Model file for the job. Use its own axes, mm. Face numbers are marked on the shaded views. A direction names the side the tool comes from. Round coordinates to 2 decimals unless told otherwise and drop trailing zeros. Order: outer loops, then holes, each group sorted by start corner. A loop starts at its lowest first (then second) coordinate and runs counter-clockwise, first axis right, second up. Notation, with made-up numbers: M 70,0.5 L 91,0.5 A16 ccw 91,30.5 Z; hole C 25.5,14.5 d1. An arc over 180 degrees is marked long. Return JSON: item names as keys, results as strings. Group by question number.
Item 1: Slice it at D-D on z = 1. Write the cut outline in (x, y), then the cut area to 3 significant figures.
Item 2: Pin check, flat tips, straight feed: pin 1 Ø8 at (y, z) = (4.5, 11) entering from -X; pin 2 Ø1.6 at (x, y) = (-0.5, -34) entering from +Z; pin 3 Ø3 at (x, z) = (0.5, 13.5) entering from +Y; pin 4 Ø12.5 at (x, y) = (-2.5, -8.5) entering from +Z. Stop position of each tip, or through.
Item 3: Which spindle directions (+Z, -Z, +X, -X, +Y, -Y) get a long thin tool onto all of the face, cutting with end or side? Do the marked faces 1, 2 and 3. Say none if no direction does.
Item 4: Slice it at C-C on y = -24.5. Write the cut outline in (x, z).
Item 5: Probe line 1 along Y through (x, z) = (5, 2.1); line 2 along Y through (x, z) = (-5, 12); line 3 along X through (y, z) = (24.5, 7.5). List the from-to ranges inside material, lowest first.
Item 6: Slice it at A-A on z = 6. Write the cut outline in (x, y).
Item 7: Pull direction Y, two halves, no side cores. Call the marked faces 4, 5 and 6: pulls with the +Y half, pulls with the -Y half, needs draft (parallel to the pull), parting line crosses it, or undercut.
Item 8: Slice it at B-B on x = 5. Give the number of separate pieces and of enclosed holes in the cut face, then the cut area to 3 significant figures.
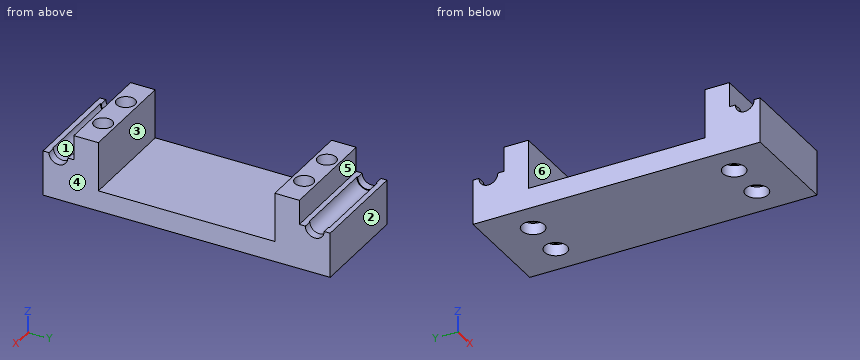
Autodesk Inventor part; units mm, degrees
ref_plane "YZ Plane" through (0, 0, 0) normal (1, 0, 0) x (0, 1, 0)
ref_plane "XZ Plane" through (0, 0, 0) normal (0, 1, 0) x (-1, 0, 0)
ref_plane "XY Plane" through (0, 0, 0) normal (0, 0, 1) x (1, 0, 0)
sketch "Sketch1" plane through (0, 0, 0) normal (0, 0, 1) x (1, 0, 0)
  line L0 (12.5, -35) -> (-12.5, -35)
  line L1 (-12.5, -35) -> (-12.5, 35)
  line L2 (-12.5, 35) -> (12.5, 35)
  line L3 (12.5, 35) -> (12.5, -35)
  line L4 (12.5, -35) -> (-12.5, 35) construction
  line L5 (-12.5, -35) -> (12.5, 35) construction
  line L6 (5, -24.5) -> (-5, -24.5) construction
  line L7 (-5, -24.5) -> (-5, 24.5) construction
  line L8 (-5, 24.5) -> (5, 24.5) construction
  line L9 (5, 24.5) -> (5, -24.5) construction
  line L10 (5, -24.5) -> (-5, 24.5) construction
  line L11 (-5, -24.5) -> (5, 24.5) construction
  circle A0 centre (-5, 24.5) radius 2.25
  circle A1 centre (5, 24.5) radius 2.25
  circle A2 centre (5, -24.5) radius 2.25
  circle A3 centre (-5, -24.5) radius 2.25
  point P0 (0, 0)
  dimension "d0" = 4.5
  dimension "d1" = 10
  dimension "d2" = 49
  dimension "d3" = 25
  dimension "d4" = 70
extrude "Extrusion1" add sketch "Sketch1" along normal blind 5
sketch "Sketch2" plane through (12.5, -35, 0) normal (1, 0, 0) x (0, 0, -1)
  line L0 (-5, 70) -> (-11, 70)
  line L1 (-11, 70) -> (-11, 62.5)
  line L2 (-11, 62.5) -> (-5, 62.5)
  line L3 (-5, 62.5) -> (-5, 70)
  circle A0 centre (-11, 66.25) radius 2.5
  line L4 (2.8141, 35) -> (-33.1304, 35) construction
  line L5 (0, 0) -> (0, 70)
  line L6 (-5, 0) -> (-11, 0)
  line L7 (-11, 0) -> (-11, 7.5)
  line L8 (-11, 7.5) -> (-5, 7.5)
  line L9 (-5, 7.5) -> (-5, 0)
  circle A1 centre (-11, 3.75) radius 2.5
  line L10 (-5, 62.5) -> (-17, 62.5)
  line L11 (-17, 62.5) -> (-17, 56.5)
  line L12 (-17, 56.5) -> (-5, 56.5)
  line L13 (-5, 56.5) -> (-5, 62.5)
  line L14 (-5, 7.5) -> (-17, 7.5)
  line L15 (-17, 7.5) -> (-17, 13.5)
  line L16 (-17, 13.5) -> (-5, 13.5)
  line L17 (-5, 13.5) -> (-5, 7.5)
  circle A2 centre (-11, 66.25) radius 2.3
  circle A3 centre (-11, 3.75) radius 2.3
  point P0 (0, 35)
  point P1 (0, 35)
  point P2 (-11, 68.75)
  point P3 (-11, 63.75)
  point P4 (-11, 6.25)
  point P5 (-11, 1.25)
  point P6 (-11, 6.05)
  point P7 (-11, 1.45)
  point P8 (-11, 68.55)
  point P9 (-11, 63.95)
  dimension "d7" = 6
  dimension "d8" = 7.5
  dimension "d9" = 5
  dimension "d12" = 6
  dimension "d13" = 12
  dimension "d16" = 0.2
extrude "Extrusion2" add sketch "Sketch2" against normal up to surface (25 mm away) contours L3 L2 L1 A0 L0 | L13 L12 L11 L10 L2 | L6 L7 A1 L8 L9 | L8 L14 L15 L16 L17
extrude "Extrusion3" cut sketch "Sketch1" along normal up to surface (17 mm away) contours A0 | A1 | A2 | A3
extrude "Extrusion4" add sketch "Sketch2" against normal blind 2 contours A0 L1 A2 | L7 A3 A1 picked at (-9.3509, 68.0205) picked at (-8.6068, 3.394)
mirror "Mirror1" about plane through (0, 0, 0) normal (1, 0, 0) of "Extrusion4"
sketch "Sketch3" plane through (0, 0, 0) normal (0, 0, -1) x (-1, 0, 0)
  circle A0 centre (-5, 24.5) radius 2.75
  circle A1 centre (-5, 24.5) radius 2.25
  line L0 (-5, 24.5) -> (-5, 16.1694) construction
  line L1 (-5, 24.5) -> (-0.8082, 24.5) construction
  circle A2 centre (-5, -24.5) radius 2.75
  circle A3 centre (5, 24.5) radius 2.75
  circle A4 centre (5, -24.5) radius 2.75
  circle A5 centre (5, 24.5) radius 2.25
  circle A6 centre (5, -24.5) radius 2.25
  circle A7 centre (-5, -24.5) radius 2.25
  point P0 (0, 0)
  dimension "d19" = 5.5
  dimension "d22" = 49
  dimension "d25" = 10
extrude "Extrusion5" cut sketch "Sketch3" against normal blind 2.8
equation "\"d13\" = 2 * d7"
equation "\"d14\" = d2"
properties part number "Servo_mount_front"
Output values:
{
 "1": {"outline": "M -12.5,-35 L 12.5,-35 L 12.5,35 L -12.5,35 Z; hole C -5,-24.5 d5.5; hole C -5,24.5 d5.5; hole C 5,-24.5 d5.5; hole C 5,24.5 d5.5", "area": "1,650 mm²"},
 "2": {"pin 1": "through", "pin 2": "z = 11", "pin 3": "y = 27.5", "pin 4": "z = 5"},
 "3": {"face 1": "+Z", "face 2": "+Z, -Z, +X, -X, +Y", "face 3": "+Z, +X, -X"},
 "4": {"outline": "M -12.5,0 L -7.75,0 L -7.75,2.8 L -7.25,2.8 L -7.25,17 L -12.5,17 Z; M -2.75,2.8 L -2.25,2.8 L -2.25,0 L 2.25,0 L 2.25,2.8 L 2.75,2.8 L 2.75,17 L -2.75,17 Z; M 7.25,2.8 L 7.75,2.8 L 7.75,0 L 12.5,0 L 12.5,17 L 7.25,17 Z"},
 "5": {"line 1": "-35 to -27.25, -21.75 to 21.75, 27.25 to 35", "line 2": "-27.5 to -26.75, -22.25 to -21.5, 21.5 to 22.25, 26.75 to 27.5", "line 3": "-12.5 to -7.25, -2.75 to 2.75, 7.25 to 12.5"},
 "6": {"outline": "M -12.5,-35 L 12.5,-35 L 12.5,-21.5 L -12.5,-21.5 Z; M -12.5,21.5 L 12.5,21.5 L 12.5,35 L -12.5,35 Z; hole C -5,-24.5 d4.5; hole C -5,24.5 d4.5; hole C 5,-24.5 d4.5; hole C 5,24.5 d4.5"},
 "7": {"face 4": "needs draft", "face 5": "pulls with the +Y half", "face 6": "undercut"},
 "8": {"separate pieces": "3", "enclosed holes": "0", "area": "406 mm²"}
}
